Geometry check sheet. Reference: the model listing, model coordinates, mm. A direction names the side the tool comes from. Give positions to 0.01 mm unless a question says otherwise; leave off trailing zeros. Loops run counter-clockwise (first coordinate to the right, second up) from the corner with the lowest first, then second, coordinate; pieces in that order, holes last. Notation, with made-up numbers: (2.5, 23) -> (25.5, 23) arc R21 cw to (25.5, 53) -> close; hole circle Ø10 at (33, -38.5). An arc over 180 degrees is marked (long way). Answer as a JSON object with one key per item and string values.
from build123d import *

# Parameters (mm, degrees)
SKETCH1_W                       = 19.05
SKETCH1_H                       = 19.05
BOSS_EXTRUDE1_DEPTH             = 25.4
SKETCH2_W                       = 6.35
SKETCH2_H                       = 6.35
CUT_EXTRUDE1_DEPTH              = 20.05
F_8_32_TAPPED_HOLE1_D           = 3.4544
F_8_32_TAPPED_HOLE1_CSINK_D     = 5.4356
F_8_32_TAPPED_HOLE1_CSINK_ANGLE = 100


with BuildPart() as part:
    # Sketch1 → Boss-Extrude1 (new body)
    with BuildSketch(Plane(origin=(0, 0, 0), x_dir=(1, 0, 0), z_dir=(0, 1, 0))):
        Rectangle(SKETCH1_W, SKETCH1_H)
    extrude(amount=BOSS_EXTRUDE1_DEPTH)

    # Sketch2 → Cut-Extrude1 (cut, through all)
    with BuildSketch(Plane.XY.offset(9.525)):
        with Locations((0, 3.175)):
            Rectangle(SKETCH2_W, SKETCH2_H)
    extrude(amount=-CUT_EXTRUDE1_DEPTH, mode=Mode.SUBTRACT)

    # #8-32 Tapped Hole1 (through all)
    with Locations(Plane(origin=(9.525, 0, 0), x_dir=(0, 0, 1), z_dir=(1, 0, 0))):
        with Locations((0, -15.875)):
            CounterSinkHole(F_8_32_TAPPED_HOLE1_D / 2, F_8_32_TAPPED_HOLE1_CSINK_D / 2, counter_sink_angle=F_8_32_TAPPED_HOLE1_CSINK_ANGLE)


solid = part.part
1) Section check A-A on y = 4.5. Record the cut outline in (x, z) (3 decimals), plus the area to 3 significant figures.
Geometry check:
{"outline": "(-9.525, -9.525) -> (-3.175, -9.525) -> (-3.175, 9.525) -> (-9.525, 9.525) -> close; (3.175, -9.525) -> (9.525, -9.525) -> (9.525, 9.525) -> (3.175, 9.525) -> close", "area": "242 mm2"}
2) Section check C-C on z = -7. Record the cut outline in (x, y) (3 decimals), plus the area to 3 significant figures.
Geometry check:
{"outline": "(-9.525, 0) -> (-3.175, 0) -> (-3.175, 6.35) -> (3.175, 6.35) -> (3.175, 0) -> (9.525, 0) -> (9.525, 25.4) -> (-9.525, 25.4) -> close", "area": "444 mm2"}
3) Draft check along X on faces 1 (the face through (-9.525, 13, 0)), 2 (the face through (0, 6.35, 0)), 3 (the face through (-0.54, 14.16, 0.22)). Enter one of: pulls with the +X half, pulls with the -X half, needs draft (parallel to the pull), parting line crosses it, or undercut.
Geometry check:
{"face 1": "pulls with the -X half", "face 2": "undercut", "face 3": "needs draft"}
4) Material ranges on line 1 along X through (y, z) = (2.75, -8) (3 decimals); line 2 along Y through (x, z) = (-1, 0); line 3 along Z through (x, y) = (8.5, 15.25) (3 decimals), recorded low to high. Write a range as from..to.
Geometry check:
{"line 1": "x = -9.525..-3.175, 3.175..9.525", "line 2": "y = 6.35..14.15, 17.6..25.4", "line 3": "z = -9.525..-1.61, 1.61..9.525"}
5) Depth check by flat-ended pin: P1, Ø3, axis at x = 0.5, z = 0.5, coming from the -Y side. Enter the tip coordinate at first touch or a pass-through.
Geometry check:
{"P1": "stops at y = 6.35"}
6) Tool access check on faces 4 (the face through (6, 0, 0)), 5 (the face through (-3.175, 3, 0)). Record the directions out of +Z, -Z, +X, -X, +Y, -Y that give a thin tool (end or side, any length) a straight path to the whole face; none if there is none.
Geometry check:
{"face 4": "+Z, -Z, +X, -X, -Y", "face 5": "+Z, -Z, -Y"}
7) Section check D-D on x = -0.75. Record the cut outline in (y, z) (3 decimals), plus the area to 3 significant figures.
Geometry check:
{"outline": "(6.35, -9.525) -> (25.4, -9.525) -> (25.4, 9.525) -> (6.35, 9.525) -> close; hole circle Ø3.454 at (15.875, 0)", "area": "354 mm2"}
8) Section check B-B on z = 0. Record the cut outline in (x, y) (3 decimals).
Geometry check:
{"outline": "(-9.525, 0) -> (-3.175, 0) -> (-3.175, 6.35) -> (3.175, 6.35) -> (3.175, 0) -> (9.525, 0) -> (9.525, 13.157) -> (8.694, 14.148) -> (-9.525, 14.148) -> close; (-9.525, 17.602) -> (8.694, 17.602) -> (9.525, 18.593) -> (9.525, 25.4) -> (-9.525, 25.4) -> close"}
